Work out the finished part from the listing and answer in its coordinate system (mm). A direction names the side the tool comes from. Round coordinates to 2 decimals unless told otherwise and drop trailing zeros. Write each loop counter-clockwise with the first axis right and the second up, starting at its lowest first coordinate (ties: lowest second). Pieces come first, ordered by that corner, then holes. Notation, with made-up numbers: (46.25, -25) - (100.25, -25) arc R11 ccw to (100.25, -17) - close; hole circle Ø2 at (-39, 25.5). An arc over 180 degrees is marked (long way). Write item = value, one per line. Start each with the question number.
from build123d import *

# Parameters (mm, degrees)
PAD_DEPTH        = 4
HOLE_D           = 3.1
HOLE_CSINK_D     = 6.3
HOLE_CSINK_ANGLE = 90
SKETCH002_R      = 1.2
HOLE001_DEPTH    = 4.001


with BuildPart() as part:
    # Sketch → Pad (new body)
    with BuildSketch(Plane.XY):
        Polygon((-13, -13), (-13, 13), (13, 13), (13, -13), (7.2, -13), (7.2, -9.5), (-7.2, -9.5), (-7.2, -13), align=None)
    extrude(amount=-PAD_DEPTH)

    # Hole (through all)
    with Locations(Plane.XY):
        with Locations((0, 0)):
            CounterSinkHole(HOLE_D / 2, HOLE_CSINK_D / 2, counter_sink_angle=HOLE_CSINK_ANGLE)

    # Sketch002 → Hole001 (cut, through all)
    with BuildSketch(Plane.XY):
        with Locations((-10.15, 10.15)):
            Circle(SKETCH002_R)
        with Locations((10.15, 10.15)):
            Circle(SKETCH002_R)
        with Locations((10.15, -10.15)):
            Circle(SKETCH002_R)
        with Locations((-10.15, -10.15)):
            Circle(SKETCH002_R)
    extrude(amount=-HOLE001_DEPTH, mode=Mode.SUBTRACT)


solid = part.part
1. Consider line 1 (Y direction, x = -10.15, z = -0.9); line 2 (X direction, y = 10, z = -1.8); line 3 (X direction, y = 0, z = -2.7). Determine where each line is inside the solid, lowest interval first.
2. Find section B-B on z = -3.45. Give the vertices of the cut face in (x, y), plus the area to 3 significant figures.
3. Which of the six approach directions +Z, -Z, +X, -X, +Y, -Y give full straight-line access (tool end or side, diameter ignored) to faces 1 (the face through (9.266, -9.339, -1.972)), 2 (the face through (-7.2, -11, -2))?
4. Find section A-A on y = 10.15. Give the vertices of the cut face in (x, z).
5. Find section D-D on y = -10.15. Give the vertices of the cut face in (x, z).
6. This flat-tipped pin is pushed along its axis until it touches: pin 1 (4 mm diameter, centred on x = 0, y = 0, fed in from +Z). Where does it stop, or does it pass through?
7. For a pull along X with two mould halves and no side action, classify faces 3 (the face through (3, 3, 0)), 4 (the face through (7.2, -11, -2)), 5 (the face through (13, 0, -2)) as released by +X, released by -X, zero draft, split by the parting line, or undercut.
Answer key:
q1.line_1 = -13 to -11.35, -8.95 to 8.95, 11.35 to 13
q1.line_2 = -13 to -11.34, -8.96 to 8.96, 11.34 to 13
q1.line_3 = -13 to -1.55, 1.55 to 13
q2.outline = (-13, -13) - (-7.2, -13) - (-7.2, -9.5) - (7.2, -9.5) - (7.2, -13) - (13, -13) - (13, 13) - (-13, 13) - close; hole circle Ø2.4 at (-10.15, -10.15); hole circle Ø2.4 at (-10.15, 10.15); hole circle Ø3.1 at (0, 0); hole circle Ø2.4 at (10.15, -10.15); hole circle Ø2.4 at (10.15, 10.15)
q2.area = 600 mm²
q3.face_1 = +Z, -Z
q3.face_2 = +Z, -Z, -Y
q4.outline = (-13, -4) - (-11.35, -4) - (-11.35, 0) - (-13, 0) - close; (-8.95, -4) - (8.95, -4) - (8.95, 0) - (-8.95, 0) - close; (11.35, -4) - (13, -4) - (13, 0) - (11.35, 0) - close
q5.outline = (-13, -4) - (-11.35, -4) - (-11.35, 0) - (-13, 0) - close; (-8.95, -4) - (-7.2, -4) - (-7.2, 0) - (-8.95, 0) - close; (7.2, -4) - (8.95, -4) - (8.95, 0) - (7.2, 0) - close; (11.35, -4) - (13, -4) - (13, 0) - (11.35, 0) - close
q6.pin_1 = -1.15
q7.face_3 = zero draft
q7.face_4 = undercut
q7.face_5 = released by +X
